```python
from build123d import *

# Parameters (mm, degrees)
F0_R     = 35
F1_DEPTH = 1
F4_D     = 6
F5_D     = 2


with BuildPart() as f1:
    # F0 (on Front) → F1 (new body)
    with BuildSketch(Plane.XZ):
        Circle(F0_R)
    extrude(amount=F1_DEPTH)

    # F4 (through all)
    with Locations(Plane.XZ.offset(4.318)):
        with Locations((-9.5, 0), (9.5, 0), (0, 0)):
            Hole(F4_D / 2)

    # F5 (through all)
    with Locations(Plane.XZ.offset(4.318)):
        with Locations((0, 7.5), (0, -7.5)):
            Hole(F5_D / 2)


solid = f1.part
```
Can you work these out from the model? Positions are in its coordinate system, mm. Give positions to 0.01 mm unless a question says otherwise; leave off trailing zeros. Loops run counter-clockwise (first coordinate to the right, second up) from the corner with the lowest first, then second, coordinate; pieces in that order, holes last. Notation, with made-up numbers: M 10,26 L 31,26 A16 cw 31,47 Z; hole C 42,59.25 d1. An arc over 180 degrees is marked long. Use one line per item in the form item = value. Start each with the question number.
(1) I want a section at C-C, the plane y = -0.55. Write out the boundary of the cut face in (x, z).
(2) I'm going to push a flat-ended pin straight in: P1, Ø2.5, axis at x = 0, z = 7.5, coming from the -Y side. Where does the tip first touch, or does it pass through?
(3) Thinking about a two-plate mould opening in X: for faces 1 (the cylindrical face through (-27.77, -0.49, -21.3)), 2 (the flat face through (7, -1, -7)), 3 (the cylindrical face through (0.13, -0.49, 8.49)), which applies, released by +X, released by -X, zero draft, split by the parting line, or undercut?
(4) I want a section at D-D, the plane z = -7.5. Write out the boundary of the cut face in (x, y), and give its area (3 significant figures).
(5) I want a section at B-B, the plane z = 0. Write out the boundary of the cut face in (x, y), and give its area (3 significant figures).
(6) I want a section at A-A, the plane x = 0. Write out the boundary of the cut face in (y, z), and give its area (3 significant figures).
(7) Please list where these lines run through material, in increasing order: line 1 (Z direction, x = 0, y = -0.5); line 2 (X direction, y = -0.9, z = 1); line 3 (Z direction, x = -12, y = -0.45).
Worked out:
q1.outline = C 0,0 d70; hole C -9.5,0 d6; hole C 0,0 d6; hole C 0,-7.5 d2; hole C 0,7.5 d2; hole C 9.5,0 d6
q2.P1 = -1
q3.face_1 = split by the parting line
q3.face_2 = zero draft
q3.face_3 = undercut
q4.outline = M -34.19,-1 L -1,-1 L -1,0 L -34.19,0 Z; M 1,-1 L 34.19,-1 L 34.19,0 L 1,0 Z
q4.area = 66.4 mm²
q5.outline = M -35,-1 L -12.5,-1 L -12.5,0 L -35,0 Z; M -6.5,-1 L -3,-1 L -3,0 L -6.5,0 Z; M 3,-1 L 6.5,-1 L 6.5,0 L 3,0 Z; M 12.5,-1 L 35,-1 L 35,0 L 12.5,0 Z
q5.area = 52.0 mm²
q6.outline = M -1,-35 L 0,-35 L 0,-8.5 L -1,-8.5 Z; M -1,-6.5 L 0,-6.5 L 0,-3 L -1,-3 Z; M -1,3 L 0,3 L 0,6.5 L -1,6.5 Z; M -1,8.5 L 0,8.5 L 0,35 L -1,35 Z
q6.area = 60.0 mm²
q7.line_1 = -35 to -8.5, -6.5 to -3, 3 to 6.5, 8.5 to 35
q7.line_2 = -34.99 to -12.33, -6.67 to -2.83, 2.83 to 6.67, 12.33 to 34.99
q7.line_3 = -32.88 to -1.66, 1.66 to 32.88
